Here's how the part is built. I have some questions about the finished solid (model axes, mm). Coordinates: 2 decimals unless noted, no trailing zeros. Order: outer loops, then holes, each group sorted by start corner. A loop starts at its lowest first (then second) coordinate and runs counter-clockwise, first axis right, second up. Notation, with made-up numbers: (17.25, 43) - (55.25, 43) arc R20 ccw to (55.25, 62) - close; hole circle Ø11 at (6.5, 51). An arc over 180 degrees is marked (long way). Use CSV: the item, a comma, the result in double quotes. Start each with the question number.
from build123d import *

# Parameters (mm, degrees)
SKETCH1_W           = 139.7
SKETCH1_H           = 50.8
BOSS_EXTRUDE1_DEPTH = 25.4
CUT_EXTRUDE1_REACH  = 146.244
SKETCH2_W           = 50.8
SKETCH2_H           = 22.225
SKETCH3_R           = 3.175
CUT_EXTRUDE2_DEPTH  = 75.392628163
SKETCH5_W           = 50.8
SKETCH5_H           = 3.175
BOSS_EXTRUDE2_DEPTH = 25.4
SKETCH7_W           = 50.8
SKETCH7_H           = 3.175
BOSS_EXTRUDE3_DEPTH = 25.4
CUT_EXTRUDE3_REACH  = 100.63
SKETCH8_R           = 3.175


with BuildPart() as part:
    # Sketch1 → Boss-Extrude1 (new body)
    with BuildSketch(Plane(origin=(0, 0, 0), x_dir=(1, 0, 0), z_dir=(0, 1, 0))):
        Rectangle(SKETCH1_W, SKETCH1_H)
    extrude(amount=BOSS_EXTRUDE1_DEPTH)

    # Sketch2 → Cut-Extrude1 (cut, up to next)
    with BuildSketch(Plane.ZY.offset(69.85), mode=Mode.PRIVATE) as cut_extrude1_sk1:
        with Locations((0, 11.1125)):
            Rectangle(SKETCH2_W, SKETCH2_H)
    cut_extrude1_tool1 = extrude(cut_extrude1_sk1.sketch, amount=-CUT_EXTRUDE1_REACH, mode=Mode.PRIVATE) & part.part
    add(cut_extrude1_tool1.solids().sort_by_distance((-69.85, 11.1125, 0))[0], mode=Mode.SUBTRACT)

    # Sketch3 → Cut-Extrude2 (cut, through all)
    with BuildSketch(Plane(origin=(0, 25.4, 0), x_dir=(1, 0, 0), z_dir=(0, 1, 0))):
        with Locations(Location((-57.15, 12.7, 0), (0, 0, 270))):
            Circle(SKETCH3_R)
        with Locations(Location((-57.15, -12.7, 0), (0, 0, 270))):
            Circle(SKETCH3_R)
        with Locations(Location((57.15, -12.7, 0), (0, 0, 270))):
            Circle(SKETCH3_R)
        with Locations(Location((57.15, 12.7, 0), (0, 0, 270))):
            Circle(SKETCH3_R)
    extrude(amount=-CUT_EXTRUDE2_DEPTH, mode=Mode.SUBTRACT)

    # Sketch5 → Boss-Extrude2 (add)
    with BuildSketch(Plane.ZY.offset(69.85)):
        with Locations((0, 23.8125)):
            Rectangle(SKETCH5_W, SKETCH5_H)
    extrude(amount=BOSS_EXTRUDE2_DEPTH)

    # Sketch7 → Boss-Extrude3 (add)
    with BuildSketch(Plane(origin=(69.85, 0, 0), x_dir=(0, 0, -1), z_dir=(1, 0, 0))):
        with Locations((0, 23.8125)):
            Rectangle(SKETCH7_W, SKETCH7_H)
    extrude(amount=BOSS_EXTRUDE3_DEPTH)

    # Sketch8 → Cut-Extrude3 (cut, up to next)
    with BuildSketch(Plane(origin=(0, 25.4, 0), x_dir=(1, 0, 0), z_dir=(0, 1, 0)), mode=Mode.PRIVATE) as cut_extrude3_sk1:
        with Locations(Location((-82.55, 12.7, 0), (0, 0, 270))):
            Circle(SKETCH8_R)
    cut_extrude3_tool1 = extrude(cut_extrude3_sk1.sketch, amount=-CUT_EXTRUDE3_REACH, mode=Mode.PRIVATE) & part.part
    # Sketch8 → Cut-Extrude3 (cut, up to next)
    with BuildSketch(Plane(origin=(0, 25.4, 0), x_dir=(1, 0, 0), z_dir=(0, 1, 0)), mode=Mode.PRIVATE) as cut_extrude3_sk2:
        with Locations(Location((-82.55, -12.7, 0), (0, 0, 270))):
            Circle(SKETCH8_R)
    cut_extrude3_tool2 = extrude(cut_extrude3_sk2.sketch, amount=-CUT_EXTRUDE3_REACH, mode=Mode.PRIVATE) & part.part
    # Sketch8 → Cut-Extrude3 (cut, up to next)
    with BuildSketch(Plane(origin=(0, 25.4, 0), x_dir=(1, 0, 0), z_dir=(0, 1, 0)), mode=Mode.PRIVATE) as cut_extrude3_sk3:
        with Locations(Location((82.55, -12.7, 0), (0, 0, 270))):
            Circle(SKETCH8_R)
    cut_extrude3_tool3 = extrude(cut_extrude3_sk3.sketch, amount=-CUT_EXTRUDE3_REACH, mode=Mode.PRIVATE) & part.part
    # Sketch8 → Cut-Extrude3 (cut, up to next)
    with BuildSketch(Plane(origin=(0, 25.4, 0), x_dir=(1, 0, 0), z_dir=(0, 1, 0)), mode=Mode.PRIVATE) as cut_extrude3_sk4:
        with Locations(Location((82.55, 12.7, 0), (0, 0, 270))):
            Circle(SKETCH8_R)
    cut_extrude3_tool4 = extrude(cut_extrude3_sk4.sketch, amount=-CUT_EXTRUDE3_REACH, mode=Mode.PRIVATE) & part.part
    add(cut_extrude3_tool1.solids().sort_by_distance((-82.55, 25.4, -12.7))[0], mode=Mode.SUBTRACT)
    add(cut_extrude3_tool2.solids().sort_by_distance((-82.55, 25.4, 12.7))[0], mode=Mode.SUBTRACT)
    add(cut_extrude3_tool3.solids().sort_by_distance((82.55, 25.4, 12.7))[0], mode=Mode.SUBTRACT)
    add(cut_extrude3_tool4.solids().sort_by_distance((82.55, 25.4, -12.7))[0], mode=Mode.SUBTRACT)


solid = part.part
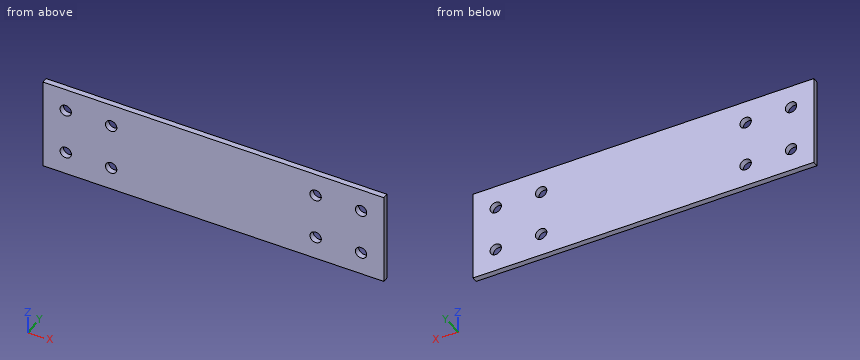
Item 1: Please list where these lines run through material, in increasing order: line 1 along X through (y, z) = (23.9, 12.7) (3 decimals); line 2 along X through (y, z) = (24.05, -12). Write a range as from..to.
Item 2: Suppose I cut it at B-B on z = 12.7. Write out the boundary of the cut face in (x, y) (3 decimals).
Item 3: Suppose I cut it at C-C on x = 57.15. Write out the boundary of the cut face in (y, z) (3 decimals), then the cut area to 3 significant figures.
Item 4: Suppose I cut it at A-A on y = 23.1. State how many separate pieces and enclosed holes the cut face has, then the cut area to 3 significant figures.
Here are the results:
1,line 1,"-95.25..-85.725, -79.375..-60.325, -53.975..53.975, 60.325..79.375, 85.725..95.25"
1,line 2,"-95.25..-85.65, -79.45..-60.25, -54.05..54.05, 60.25..79.45, 85.65..95.25"
2,outline,"(-95.25, 22.225) - (-85.725, 22.225) - (-85.725, 25.4) - (-95.25, 25.4) - close; (-79.375, 22.225) - (-60.325, 22.225) - (-60.325, 25.4) - (-79.375, 25.4) - close; (-53.975, 22.225) - (53.975, 22.225) - (53.975, 25.4) - (-53.975, 25.4) - close; (60.325, 22.225) - (79.375, 22.225) - (79.375, 25.4) - (60.325, 25.4) - close; (85.725, 22.225) - (95.25, 22.225) - (95.25, 25.4) - (85.725, 25.4) - close"
3,outline,"(22.225, -25.4) - (25.4, -25.4) - (25.4, -15.875) - (22.225, -15.875) - close; (22.225, -9.525) - (25.4, -9.525) - (25.4, 9.525) - (22.225, 9.525) - close; (22.225, 15.875) - (25.4, 15.875) - (25.4, 25.4) - (22.225, 25.4) - close"
3,area,"121 mm^2"
4,separate pieces,"1"
4,enclosed holes,"8"
4,area,"9,420 mm^2"
